from build123d import *

# Parameters (mm, degrees)
SZKIC1_W                    = 180
SZKIC1_H                    = 240
DODANIE_WYCI_GNI_CIE1_DEPTH = 5
SZKIC2_R                    = 57.5
SZKIC2_R_2                  = 4.25
WYTNIJ_WYCI_GNI_CIE1_DEPTH  = 43
SZYK_KO_OWY1_COUNT          = 4


with BuildPart() as part:
    # Szkic1 → Dodanie-wyciągnięcie1 (new body)
    with BuildSketch(Plane(origin=(0, 0, 0), x_dir=(1, 0, 0), z_dir=(0, 1, 0))):
        Rectangle(SZKIC1_W, SZKIC1_H)
    extrude(amount=DODANIE_WYCI_GNI_CIE1_DEPTH)

    # Szkic2 → Wytnij-wyciągnięcie1 (cut)
    with BuildSketch(Plane(origin=(0, 0, 0), x_dir=(1, 0, 0), z_dir=(0, 1, 0))):
        Circle(SZKIC2_R)
        with Locations((0, 74.6)):
            Circle(SZKIC2_R_2)
    wytnij_wyci_gni_cie1 = extrude(amount=WYTNIJ_WYCI_GNI_CIE1_DEPTH, mode=Mode.SUBTRACT)

    # Szyk kołowy1: Wytnij-wyciągnięcie1 ×4 about axis
    szyk_ko_owy1_axis = Axis((0, 0, 0), (0, 1, 0))
    for i in range(1, SZYK_KO_OWY1_COUNT):
        add(wytnij_wyci_gni_cie1.rotate(szyk_ko_owy1_axis, i * 360 / SZYK_KO_OWY1_COUNT), mode=Mode.SUBTRACT)


solid = part.part
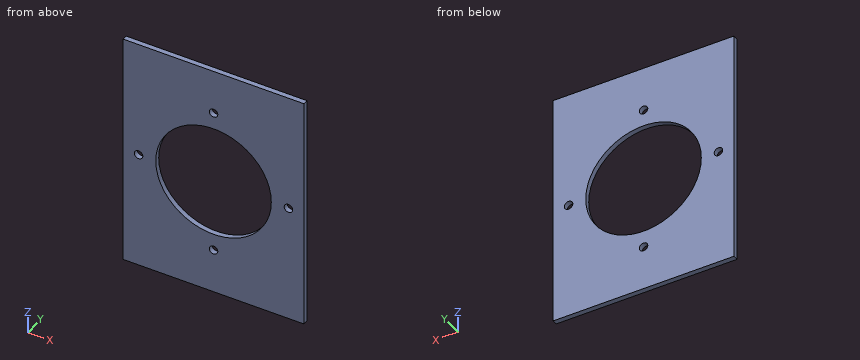
The model under review builds one solid part; all positions refer to its coordinate system, in mm. Round coordinates to 2 decimals unless told otherwise and drop trailing zeros. Loops run counter-clockwise (first coordinate to the right, second up) from the corner with the lowest first, then second, coordinate; pieces in that order, holes last. Notation, with made-up numbers: (-40, 7) - (-6, 7) arc R26 ccw to (-6, 26) - close; hole circle Ø2 at (86, 85). An arc over 180 degrees is marked (long way). Use CSV: the item, a comma, the result in double quotes.
(1) Take a section at A-A, the plane x = 0. Give the boundary of the cut face in (y, z).
Working result:
outline,"(0, -120) - (5, -120) - (5, -78.85) - (0, -78.85) - close; (0, -70.35) - (5, -70.35) - (5, -57.5) - (0, -57.5) - close; (0, 57.5) - (5, 57.5) - (5, 70.35) - (0, 70.35) - close; (0, 78.85) - (5, 78.85) - (5, 120) - (0, 120) - close"
(2) Take a section at B-B, the plane z = 0. Give the boundary of the cut face in (x, y).
Working result:
outline,"(-90, 0) - (-78.85, 0) - (-78.85, 5) - (-90, 5) - close; (-70.35, 0) - (-57.5, 0) - (-57.5, 5) - (-70.35, 5) - close; (57.5, 0) - (70.35, 0) - (70.35, 5) - (57.5, 5) - close; (78.85, 0) - (90, 0) - (90, 5) - (78.85, 5) - close"
(3) Clearance check with a flat-ended pin moving along its axis: P1, Ø7.5, axis at x = 74.6, z = 0, coming from the -Y side. State where the tip first meets the part, or that it passes through.
Working result:
P1,"passes through"
(4) Take a section at C-C, the plane x = 74.6. Give the boundary of the cut face in (y, z), plus the area to 3 significant figures.
Working result:
outline,"(0, -120) - (5, -120) - (5, -4.25) - (0, -4.25) - close; (0, 4.25) - (5, 4.25) - (5, 120) - (0, 120) - close"
area,"1,160 mm^2"
(5) For line 1 (Z direction, x = 0, y = 2.8); line 2 (X direction, y = 2.45, z = 0); line 3 (Z direction, x = 25, y = 3.8), list the stretches that pass through material, from the lowest coordinate up.
Working result:
line 1,"z = -120 to -78.85, -70.35 to -57.5, 57.5 to 70.35, 78.85 to 120"
line 2,"x = -90 to -78.85, -70.35 to -57.5, 57.5 to 70.35, 78.85 to 90"
line 3,"z = -120 to -51.78, 51.78 to 120"
(6) Take a section at D-D, the plane y = 2.9. Give the boundary of the cut face in (x, z), plus the area to 3 significant figures.
Working result:
outline,"(-90, -120) - (90, -120) - (90, 120) - (-90, 120) - close; hole circle Ø8.5 at (-74.6, 0); hole circle Ø115 at (0, 0); hole circle Ø8.5 at (0, -74.6); hole circle Ø8.5 at (0, 74.6); hole circle Ø8.5 at (74.6, 0)"
area,"32,600 mm^2"
